Geometry check sheet. Reference: drawing and pictorial views, mm from the part's lowest x, y, z. A direction names the side the tool comes from. Give positions to 0.01 mm unless a question says otherwise; leave off trailing zeros. Write each loop counter-clockwise with the first axis right and the second up, starting at its lowest first coordinate (ties: lowest second). Pieces come first, ordered by that corner, then holes. Notation, with made-up numbers: (-27.5, 40) -> (18.5, 40) arc R17 cw to (18.5, 47) -> close; hole circle Ø8 at (-23, -28.5). An arc over 180 degrees is marked (long way). Return JSON: item names as keys, results as strings.
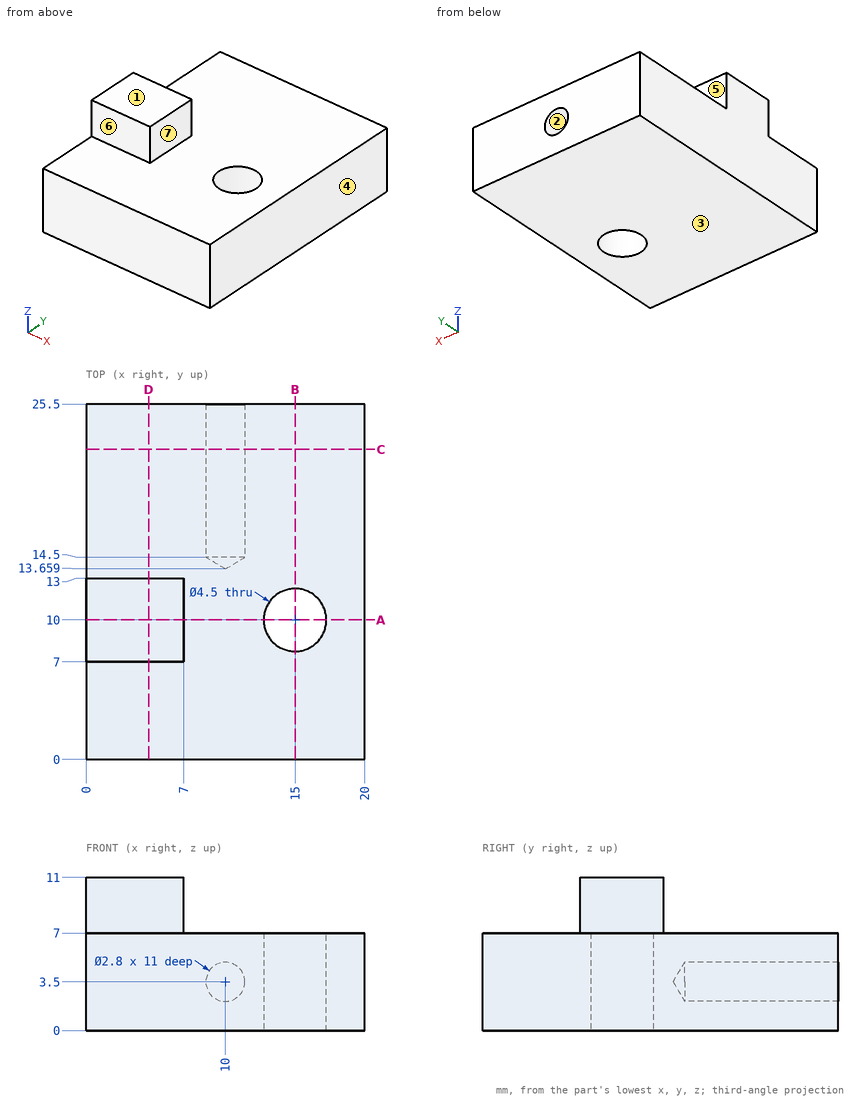
(1) Cross-section at D-D on x = 4.5. Enter the section's corners in (y, z).
Reply:
{"outline": "(0, 0) -> (25.5, 0) -> (25.5, 7) -> (13, 7) -> (13, 11) -> (7, 11) -> (7, 7) -> (0, 7) -> close"}
(2) Release check for a two-part mould opening along Z. For the marked faces 1, 2, 3 and 4 record: pulls with the +Z half, pulls with the -Z half, needs draft (parallel to the pull), parting line crosses it, or undercut.
Reply:
{"face 1": "pulls with the +Z half", "face 2": "undercut", "face 3": "pulls with the -Z half", "face 4": "needs draft"}
(3) Cross-section at C-C on y = 22.25. Enter the section's corners in (x, z).
Reply:
{"outline": "(0, 0) -> (20, 0) -> (20, 7) -> (0, 7) -> close; hole circle Ø2.8 at (10, 3.5)"}
(4) Thickness scan on L1, parallel to Z at x = 10, y = 18.75; L2, parallel to Y at x = 5, z = 8.25; L3, parallel to X at y = 10, z = 9.25. Record the ranges inside material, lowest first.
Reply:
{"L1": "0 to 2.1, 4.9 to 7", "L2": "7 to 13", "L3": "0 to 7"}
(5) Cross-section at B-B on x = 15. Enter the section's corners in (y, z).
Reply:
{"outline": "(0, 0) -> (7.75, 0) -> (7.75, 7) -> (0, 7) -> close; (12.25, 0) -> (25.5, 0) -> (25.5, 7) -> (12.25, 7) -> close"}
(6) Depth check by flat-ended pin: pin 1 Ø1.5 at (x, y) = (4, 21) entering from +Z; pin 2 Ø3 at (x, z) = (17.5, 9.5) entering from +Y; pin 3 Ø1.2 at (y, z) = (9, 9.5) entering from +X; pin 4 Ø4 at (x, z) = (6.5, 9.5) entering from +Y. Enter the tip coordinate at first touch or a pass-through.
Reply:
{"pin 1": "z = 7", "pin 2": "through", "pin 3": "x = 7", "pin 4": "y = 13"}
(7) Cross-section at A-A on y = 10. Enter the section's corners in (x, z).
Reply:
{"outline": "(0, 0) -> (12.75, 0) -> (12.75, 7) -> (7, 7) -> (7, 11) -> (0, 11) -> close; (17.25, 0) -> (20, 0) -> (20, 7) -> (17.25, 7) -> close"}
(8) Set-up check for the marked faces 5, 6 and 7: record each of +Z, -Z, +X, -X, +Y, -Y from which the full face is reachable in a straight line by a thin tool's end or side.
Reply:
{"face 5": "+Z, +X, -X, +Y", "face 6": "+Z, +X, -X, -Y", "face 7": "+Z, +X, +Y, -Y"}
